from build123d import *

# Parameters (mm, degrees)
BOSS_EXTRUDE1_DEPTH = 1.5
SKETCH2_R           = 3.75
BOSS_EXTRUDE2_DEPTH = 2.5


with BuildPart() as part:
    # Sketch1 → Boss-Extrude1 (new body)
    with BuildSketch(Plane(origin=(0, 4, 0), x_dir=(1, 0, 0), z_dir=(0, 1, 0))):
        with BuildLine():
            Line((2.25, -3), (4.407767894, -2.817669075))
            Line((4.407767894, -2.817669075), (4.407767894, 2.817669075))
            Line((4.407767894, 2.817669075), (2.25, 3))
            ThreePointArc((2.25, 3), (-3.75, 0), (2.25, -3))
        make_face()
    extrude(amount=-BOSS_EXTRUDE1_DEPTH)

    # Sketch2 → Boss-Extrude2 (add)
    with BuildSketch(Plane.XZ.offset(-2.5)):
        Circle(SKETCH2_R)
    extrude(amount=BOSS_EXTRUDE2_DEPTH)

    # Sketch3 → Cut-Revolve1 (revolve, cut)
    with BuildSketch(Plane(origin=(0, 0, 0), x_dir=(-1, 0, 0), z_dir=(0, 0, -1))):
        Polygon((-2.3, 0), (0, 0), (0, 4), (-2.3, 4), (-2.3, 3), (-1.25, 3), (-1.25, 2.5), (-2.3, 2.5), align=None)
    revolve(axis=Axis((0, 0, 0), (0, 1, 0)), mode=Mode.SUBTRACT)


solid = part.part
Verification items for the finished model (mm, model axes). A direction names the side the tool comes from. Give positions to 0.01 mm unless a question says otherwise; leave off trailing zeros. Loops run counter-clockwise (first coordinate to the right, second up) from the corner with the lowest first, then second, coordinate; pieces in that order, holes last.
1) Thickness scan on line 1 along X through (y, z) = (3.6, 0); line 2 along X through (y, z) = (2.75, 0); line 3 along Z through (x, y) = (0, 2.6). Record the ranges inside material, lowest first.
2) Sectioned sample at C-C, the plane y = 3.75. Enter the section's corners in (x, z).
3) Sectioned sample at D-D, the plane y = 2.75. Enter the section's corners in (x, z).
4) Set-up check for faces 1 (the flat face through (2, 4, -2)), 2 (the cylindrical face through (-0.27, 2.75, 1.22)), 3 (the cylindrical face through (-1.825, 1.232, 1.4)), 4 (the flat face through (4, 2.5, 0)), 5 (the flat face through (1, 3, 1)): record each of +Z, -Z, +X, -X, +Y, -Y from which the full face is reachable in a straight line by a thin tool's end or side.
5) Sectioned sample at B-B, the plane x = 0. Enter the section's corners in (y, z).
6) Sectioned sample at A-A, the plane z = 0. Enter the section's corners in (x, y), then the cut area to 3 significant figures.
7) Depth check by flat-ended pin: pin 1 Ø3.5 at (x, z) = (0, 0) entering from +Y; pin 2 Ø2 at (y, z) = (0.5, -2) entering from +X; pin 3 Ø0.6 at (x, z) = (3.5, 1.5) entering from -Y; pin 4 Ø2.5 at (x, z) = (0.5, 0) entering from -Y. Enter the tip coordinate at first touch or a pass-through.
8) Draft check along X on faces 6 (the flat face through (3.344, 3.26, -2.908)), 7 (the flat face through (2, 0, 2)), 8 (the cylindrical face through (-1.825, 3.493, 1.4)). Enter one of: pulls with the +X half, pulls with the -X half, needs draft (parallel to the pull), parting line crosses it, or undercut.
Answers:
1. line 1: x = -3.75 to -2.3, 2.3 to 4.41
1. line 2: x = -3.75 to -1.25, 1.25 to 4.41
1. line 3: z = -3.75 to -1.25, 1.25 to 3.75
2. outline: (2.25, -3) - (4.41, -2.82) - (4.41, 2.82) - (2.25, 3) arc R3.75 ccw (long way) to start; hole circle Ø4.6 at (0, 0)
3. outline: (2.25, -3) - (4.41, -2.82) - (4.41, 2.82) - (2.25, 3) arc R3.75 ccw (long way) to start; hole circle Ø2.5 at (0, 0)
4. face 1: +Z, -Z, +X, -X, +Y
4. face 2: +Y, -Y
4. face 3: -Y
4. face 4: +X, -Y
4. face 5: +Y
5. outline: (0, -3.75) - (4, -3.75) - (4, -2.3) - (3, -2.3) - (3, -1.25) - (2.5, -1.25) - (2.5, -2.3) - (0, -2.3) - close; (0, 2.3) - (2.5, 2.3) - (2.5, 1.25) - (3, 1.25) - (3, 2.3) - (4, 2.3) - (4, 3.75) - (0, 3.75) - close
6. outline: (-3.75, 0) - (-2.3, 0) - (-2.3, 2.5) - (-1.25, 2.5) - (-1.25, 3) - (-2.3, 3) - (-2.3, 4) - (-3.75, 4) - close; (1.25, 2.5) - (2.3, 2.5) - (2.3, 0) - (3.75, 0) - (3.75, 2.5) - (4.41, 2.5) - (4.41, 4) - (2.3, 4) - (2.3, 3) - (1.25, 3) - close
6. area: 13.6 mm2
7. pin 1: stops at y = 3
7. pin 2: stops at x = 3.61
7. pin 3: stops at y = 0
7. pin 4: stops at y = 2.5
8. face 6: pulls with the +X half
8. face 7: needs draft
8. face 8: undercut
